Verification items for this drawing (mm, ordinates from the low corner). Give positions to 0.01 mm unless a question says otherwise; leave off trailing zeros. Loops run counter-clockwise (first coordinate to the right, second up) from the corner with the lowest first, then second, coordinate; pieces in that order, holes last. Notation, with made-up numbers: (58.25, 14.25) -> (66.25, 14.25) arc R27 cw to (66.25, 40.25) -> close; hole circle Ø3 at (-3.75, 13.5). An arc over 180 degrees is marked (long way). Use one line per item in the form item = value. Start each with the question number.
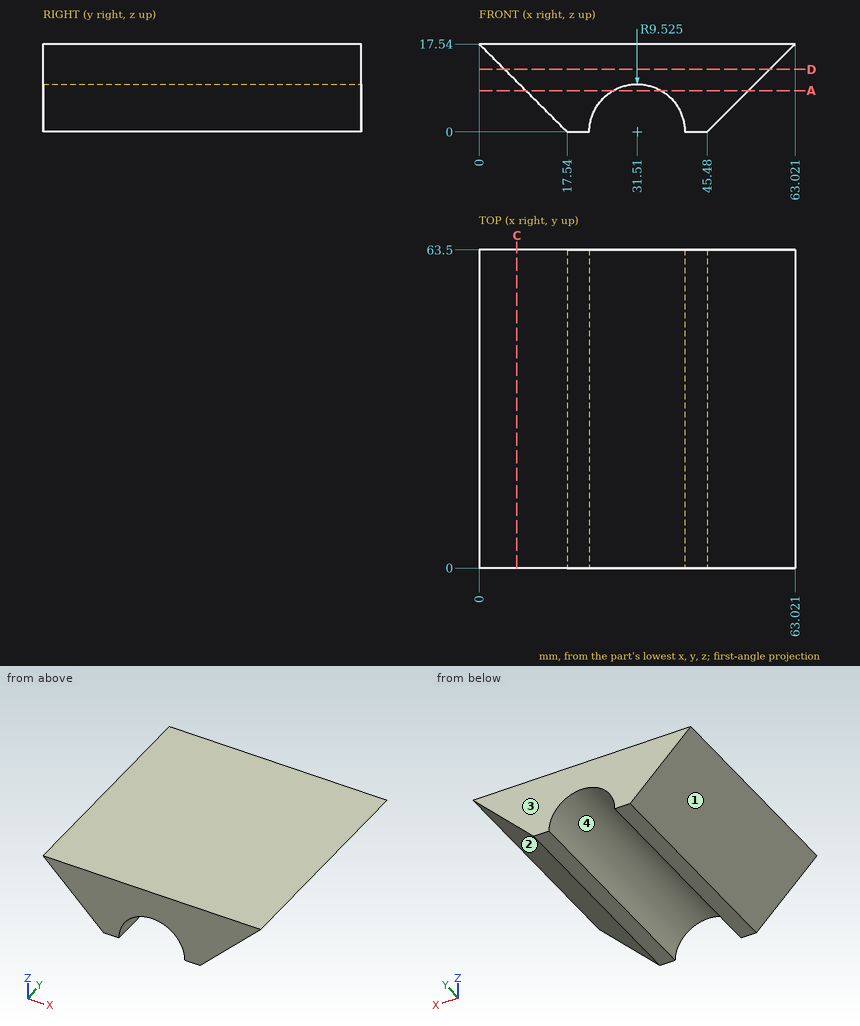
Item 1: Gauge pin test, flat ends, axial feed: pin 1 Ø1 at (y, z) = (24.5, 10.5) entering from +X; pin 2 Ø6 at (y, z) = (11, 11) entering from -X; pin 3 Ø1 at (x, y) = (8.5, 48.5) entering from -Z. Record the tip position at first contact, or that the pin passes through.
Item 2: Draft check along X on the marked faces 1, 2, 3 and 4. Enter one of: +X half, -X half, draft (parallel to the pull), parting line (faces both ways), or undercut.
Item 3: Material ranges on line 1 (X direction, y = 15, z = 3); line 2 (X direction, y = 4.5, z = 2) (1 decimal); line 3 (X direction, y = 55, z = 16.25), recorded low to high.
Item 4: Sectioned sample at D-D, the plane z = 12.5. Enter the section's corners in (x, y).
Item 5: Sectioned sample at A-A, the plane z = 8.25. Enter the section's corners in (x, y), and give its area (3 significant figures).
Item 6: Sectioned sample at C-C, the plane x = 7.5. Enter the section's corners in (y, z).
Outcome:
q1.pin_1 = 56.48
q1.pin_2 = 3.54
q1.pin_3 = 8.54
q2.face_1 = -X half
q2.face_2 = +X half
q2.face_3 = draft
q2.face_4 = undercut
q3.line_1 = 14.54 to 22.47, 40.55 to 48.48
q3.line_2 = 15.5 to 22.2, 40.8 to 47.5
q3.line_3 = 1.29 to 61.73
q4.outline = (5.04, 0) -> (57.98, 0) -> (57.98, 63.5) -> (5.04, 63.5) -> close
q5.outline = (9.29, 0) -> (26.75, 0) -> (26.75, 63.5) -> (9.29, 63.5) -> close; (36.27, 0) -> (53.73, 0) -> (53.73, 63.5) -> (36.27, 63.5) -> close
q5.area = 2,220 mm^2
q6.outline = (0, 10.04) -> (63.5, 10.04) -> (63.5, 17.54) -> (0, 17.54) -> close
